```python
from build123d import *

# Parameters (mm, degrees)
F0_R     = 115
F0_R_2   = 70
F1_DEPTH = 5
F2_R     = 8
F3_DEPTH = 25


with BuildPart() as f1:
    # F0 (on Top) → F1 (new body)
    with BuildSketch(Plane.XY):
        Circle(F0_R)
        Circle(F0_R_2, mode=Mode.SUBTRACT)
    extrude(amount=F1_DEPTH)

    # F2 (on face) → F3 (cut)
    with BuildSketch(Plane.XY.offset(5)):
        with Locations((0, 92.5)):
            Circle(F2_R)
        Polygon((30.7451541874, 84.0570025344), (42.1222582105, 72.9578913502), (50.5819233456, 64.7049331524), (57.422922467, 91.5601138634), align=None)
        Polygon((68.8072985361, 45.6942659799), (72.8301810847, 42.0485246544), (80.6630838702, 34.949948686), (91.4074011641, 46.8057340201), (79.55161583, 57.550051314), align=None)
        Polygon((100.5, -5.812340224), (100.5, 5.812340224), (89.44427191, 9.4045640367), (82.61145618, 0), (89.44427191, -9.4045640367), align=None)
        Polygon((78.6682453406, -55.374818439), (87.2901221684, -52.0587102834), (88.7292266779, -42.9338918444), (81.5464543596, -37.125181561), (72.9245775317, -40.4412897166), (71.4854730222, -49.5661081556), align=None)
        Polygon((42.3974030495, -88.1073498501), (50.1025969505, -88.1073498501), (54.906706769, -82.0831866798), (53.1921398259, -74.571178077), (46.25, -71.2280197367), (39.3078601741, -74.571178077), (37.593293231, -82.0831866798), align=None)
        Polygon((3.065005288, -99.899577335), (5.8217626423, -98.9099722116), (6.010291359, -98.510291359), align=None)
        Polygon((0.4159269752, -101.1491426608), (3.065005288, -99.899577335), (0, -100.9998355537), align=None)
        Polygon((0, -100.9998355537), (3.065005288, -99.899577335), (6.010291359, -98.510291359), (7.399577335, -95.565005288), (8.4998355537, -92.5), (7.399577335, -89.434994712), (6.010291359, -86.489708641), (3.065005288, -85.100422665), (0, -84.0001644463), (-3.065005288, -85.100422665), (-6.010291359, -86.489708641), (-7.399577335, -89.434994712), (-8.4998355537, -92.5), (-7.399577335, -95.565005288), (-6.010291359, -98.510291359), (-3.065005288, -99.899577335), align=None)
        Polygon((7.399577335, -95.565005288), (6.010291359, -98.510291359), (6.4099722116, -98.3217626423), align=None)
        Polygon((-0.4159269752, -101.1491426608), (0, -100.9998355537), (-3.065005288, -99.899577335), align=None)
        Polygon((8.4998355537, -92.5), (7.399577335, -95.565005288), (8.6491426608, -92.9159269752), align=None)
        Polygon((-5.8217626423, -98.9099722116), (-3.065005288, -99.899577335), (-6.010291359, -98.510291359), align=None)
        Polygon((7.399577335, -89.434994712), (8.4998355537, -92.5), (8.6491426608, -92.0840730248), align=None)
        Polygon((-6.4099722116, -98.3217626423), (-6.010291359, -98.510291359), (-7.399577335, -95.565005288), align=None)
        Polygon((6.010291359, -86.489708641), (7.399577335, -89.434994712), (6.4099722116, -86.6782373577), align=None)
        Polygon((-8.6491426608, -92.9159269752), (-7.399577335, -95.565005288), (-8.4998355537, -92.5), align=None)
        Polygon((3.065005288, -85.100422665), (6.010291359, -86.489708641), (5.8217626423, -86.0900277884), align=None)
        Polygon((-8.6491426608, -92.0840730248), (-8.4998355537, -92.5), (-7.399577335, -89.434994712), align=None)
        Polygon((0, -84.0001644463), (3.065005288, -85.100422665), (0.4159269752, -83.8508573392), align=None)
        Polygon((-6.4099722116, -86.6782373577), (-7.399577335, -89.434994712), (-6.010291359, -86.489708641), align=None)
        Polygon((-3.065005288, -85.100422665), (0, -84.0001644463), (-0.4159269752, -83.8508573392), align=None)
        Polygon((-5.8217626423, -86.0900277884), (-6.010291359, -86.489708641), (-3.065005288, -85.100422665), align=None)
        Polygon((-57.422922467, 91.5601138634), (-50.5819233456, 64.7049331524), (-30.7451541874, 84.0570025344), align=None)
        Polygon((-80.6630838702, 34.949948686), (-68.8072985361, 45.6942659799), (-79.55161583, 57.550051314), (-91.4074011641, 46.8057340201), align=None)
        Polygon((-100.5, -5.812340224), (-89.44427191, -9.4045640367), (-82.61145618, 0), (-89.44427191, 9.4045640367), (-100.5, 5.812340224), align=None)
        Polygon((-71.4854730222, -49.5661081556), (-72.9245775317, -40.4412897166), (-81.5464543596, -37.125181561), (-88.7292266779, -42.9338918444), (-87.2901221684, -52.0587102834), (-78.6682453406, -55.374818439), align=None)
        Polygon((-50.1025969505, -88.1073498501), (-42.3974030495, -88.1073498501), (-37.593293231, -82.0831866798), (-39.3078601741, -74.571178077), (-46.25, -71.2280197367), (-53.1921398259, -74.571178077), (-54.906706769, -82.0831866798), align=None)
    extrude(amount=-F3_DEPTH, mode=Mode.SUBTRACT)


solid = f1.part
```
The model under review builds one solid part; all positions refer to its coordinate system, in mm. A direction names the side the tool comes from. Round coordinates to 2 decimals unless told otherwise and drop trailing zeros. Loops run counter-clockwise (first coordinate to the right, second up) from the corner with the lowest first, then second, coordinate; pieces in that order, holes last. Notation, with made-up numbers: (59, 69) - (89, 69) arc R27 ccw to (89, 102) - close; hole circle Ø2 at (11, 24). An arc over 180 degrees is marked (long way). Use a Markdown table: item, result. Add a question column.
Q1. Machinability: for faces 3 (the face through (54.06, -78.38, 2.54)), 4 (the face through (50, -50, 0)), which of the approach directions +Z, -Z, +X, -X, +Y, -Y give a long, thin tool a straight path to every point of the face, cutting with its end or side? Answer none if there is none.
Q2. The part is to be moulded in two halves that separate along X. For faces 1 (the face through (50, -50, 5)), 2 (the face through (88, -47.56, 2.54)), say which applies: pulls with the +X half, pulls with the -X half, needs draft (parallel to the pull), parting line crosses it, or undercut.
Q3. For probe 1 along Y at (x, z) = (0, 2.95); probe 2 along Y at (x, z) = (-49, 2.85); probe 3 along Y at (x, z) = (75, 3.1), list the stretches that pass through material, from the lowest coordinate up.
Q4. Insertion check: pin 1 Ø2 at (y, z) = (-78, 2.5) entering from +X; pin 2 Ø9.5 at (x, y) = (0, 92.5) entering from +Z; pin 3 Ø3 at (y, z) = (-32.5, 1) entering from -X; pin 4 Ø1.5 at (x, z) = (-37, 3) entering from -Y. Each pin has a flat end and moves straight along its axis. Give the tip position at first contact, or say it passes through.
Q5. Add section A-A (x = 62.5). State the section outline as (y, z) points, plus the area to 3 significant figures.
Q6. Add section B-B (z = 4.2). State how many separate pieces and enclosed holes the cut face has, plus the area to 3 significant figures.
Worked answers:
| question | item | result |
|---|---|---|
| 1 | face 3 | +Z, -Z |
| 1 | face 4 | -Z, +X, -X, +Y, -Y |
| 2 | face 1 | needs draft |
| 2 | face 2 | undercut |
| 3 | probe 1 | -115 to -101, -84 to -70, 70 to 84.5, 100.5 to 115 |
| 3 | probe 2 | -104.04 to -88.11, -72.55 to -49.99, 49.99 to 66.25, 89.19 to 104.04 |
| 3 | probe 3 | -87.18 to -52.41, -39.64 to 40.08, 52.53 to 87.18 |
| 4 | pin 1 | x = 85.42 |
| 4 | pin 2 | through |
| 4 | pin 3 | x = -110.74 |
| 4 | pin 4 | y = -109.14 |
| 5 | outline | (-96.53, 0) - (-31.52, 0) - (-31.52, 5) - (-96.53, 5) - close; (31.52, 0) - (96.53, 0) - (96.53, 5) - (31.52, 5) - close |
| 5 | area | 650 mm² |
| 6 | separate pieces | 1 |
| 6 | enclosed holes | 13 |
| 6 | area | 23,200 mm² |
